from build123d import *

# Parameters (mm, degrees)
F_6_0_204_DIAMETER_HOLE1_D     = 5.1816
F_6_0_204_DIAMETER_HOLE1_DEPTH = 10
F_6_0_204_DIAMETER_HOLE1_TIP   = 1.556709692


with BuildPart() as part:
    # Sketch1 → Revolve1 (revolve)
    with BuildSketch(Plane.XY):
        Polygon((0, 0), (-5.55, 0), (-5.55, 79.37), (-3.55, 83.37), (-2.5, 83.37), (-2.5, 85.92), (0, 85.92), align=None)
    revolve(axis=Axis((0, 90.216, 0), (0, -1, 0)))

    # #6 (0.204) Diameter Hole1
    with Locations(Plane.XZ):
        with Locations((0, 0)):
            Hole(F_6_0_204_DIAMETER_HOLE1_D / 2, depth=F_6_0_204_DIAMETER_HOLE1_DEPTH)
            with Locations((0, 0, -(F_6_0_204_DIAMETER_HOLE1_DEPTH + F_6_0_204_DIAMETER_HOLE1_TIP / 2))):  # 118° drill point
                Cone(0, F_6_0_204_DIAMETER_HOLE1_D / 2, F_6_0_204_DIAMETER_HOLE1_TIP, mode=Mode.SUBTRACT)


solid = part.part
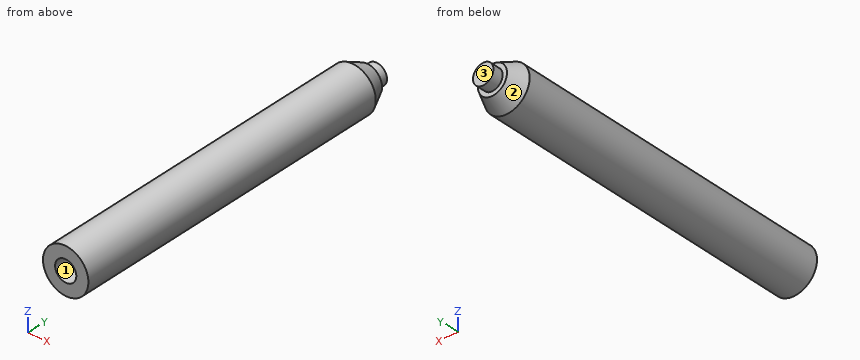
Here's how the part is built. I have some questions about the finished solid (model axes, mm). Face numbers are marked on the shaded views. Coordinates: 2 decimals unless noted, no trailing zeros. Write each loop counter-clockwise with the first axis right and the second up, starting at its lowest first coordinate (ties: lowest second). Pieces come first, ordered by that corner, then holes.
Item 1: I want a section at A-A on y = 21.5. Write out the boundary of the cut face in (x, z).
Item 2: If we mould it in two halves opening along Z, with no side actions, what happens to the marked faces 1, 2 and 3? For each: +Z half, -Z half, draft (parallel to the pull), parting line (faces both ways), or undercut.
Item 3: If I drill on line 1 (X direction, y = 6.75, z = 0); line 2 (Y direction, x = -2.25, z = -1.75), over which ranges is the centre line in solid material (lowest first)?
Item 4: Will these pins go through, and if not, where does the flat tip stop? pin 1 (1.5 mm diameter, centred on x = 0, z = -1, fed in from -Y); pin 2 (2 mm diameter, centred on y = 76.5, z = -1.5, fed in from -X); pin 3 (6 mm diameter, centred on x = 0, z = 0, fed in from -Y); pin 4 (3 mm diameter, centred on x = -3.5, y = 52, fed in from -Z).
Findings below:
1. outline: circle Ø11.1 at (0, 0)
2. face 1: undercut
2. face 2: parting line
2. face 3: draft
3. line 1: x = -5.55 to -2.59, 2.59 to 5.55
3. line 2: y = 0 to 83.37
4. pin 1: stops at y = 10.51
4. pin 2: stops at x = -5.53
4. pin 3: stops at y = 0
4. pin 4: stops at z = -5.18
